from build123d import *

# Parameters (mm, degrees)
SKETCH1_W           = 150
SKETCH1_H           = 13
BOSS_EXTRUDE1_DEPTH = 40
CUT_EXTRUDE1_DEPTH  = 40
CUT_EXTRUDE3_DEPTH  = 86.988371307
SKETCH8_R           = 2
CUT_EXTRUDE7_DEPTH  = 6.5
SKETCH4_W           = 40
SKETCH4_H           = 13
CUT_EXTRUDE10_DEPTH = 77.299594056


with BuildPart() as part:
    # Sketch1 → Boss-Extrude1 (new body)
    with BuildSketch(Plane.XY):
        Rectangle(SKETCH1_W, SKETCH1_H)
    extrude(amount=BOSS_EXTRUDE1_DEPTH)

    # Sketch2 → Cut-Extrude1 (cut)
    with BuildSketch(Plane.XZ.offset(6.5)):
        Polygon((-75, 9.270509831), (-46.468304511, 0), (-75, 0), align=None)
    extrude(amount=-CUT_EXTRUDE1_DEPTH, mode=Mode.SUBTRACT)

    # Sketch3 → Cut-Extrude3 (cut, through all)
    with BuildSketch(Plane.XZ.offset(6.5)):
        Polygon((-75, 12.424896504), (-45.99315119, 3), (75, 3), (75, 40), (-75, 40), align=None)
    extrude(amount=-CUT_EXTRUDE3_DEPTH, mode=Mode.SUBTRACT)

    # Sketch8 → Cut-Extrude7 (cut)
    with BuildSketch(Plane(origin=(-4.437328231, 0, -13.656692045), x_dir=(-0.9510565162951532, 0, 0.30901699437494873), z_dir=(-0.30901699437494873, 0, -0.9510565162951532))):
        with Locations((59.193983807, 0)):
            Circle(SKETCH8_R)
    extrude(amount=-CUT_EXTRUDE7_DEPTH, mode=Mode.SUBTRACT)

    # Sketch4 → Cut-Extrude10 (cut, through all)
    with BuildSketch(Plane.XY):
        with Locations((55, 0)):
            Rectangle(SKETCH4_W, SKETCH4_H)
    extrude(amount=CUT_EXTRUDE10_DEPTH, mode=Mode.SUBTRACT)


solid = part.part
Design review of the part built by this model. Coordinates are the model's own, in mm. A direction names the side the tool comes from. Round coordinates to 2 decimals unless told otherwise and drop trailing zeros. Write each loop counter-clockwise with the first axis right and the second up, starting at its lowest first coordinate (ties: lowest second). Pieces come first, ordered by that corner, then holes.
Item 1: For faces 1 (the flat face through (-6, 0, 3)), 2 (the flat face through (-60.93, -2.98, 4.7)), list the 3-axis set-ups (+Z, -Z, +X, -X, +Y, -Y) from which the entire face can be reached by the end or side of a thin tool; tool diameter is ignored.
Item 2: For pin 1 Ø4 at (x, z) = (-57.5, 9.5) entering from +Y; pin 2 Ø6 at (x, y) = (9.5, 2.5) entering from -Z, all flat-tipped, find the tip position at first contact; note any pin that passes through.
Item 3: Consider section B-B on x = 13. Give the boundary of the cut face in (y, z), and give its area (3 significant figures).
Item 4: Consider section C-C on z = 10.5. Give the boundary of the cut face in (x, y), and give its area (3 significant figures).
Item 5: Wall thickness on L1, parallel to Z at x = 0, y = -0.25; L2, parallel to Z at x = -54, y = 4.5: over which ranges is each line inside the solid? List them lowest first.
Item 6: Consider section A-A on y = -4.5. Give the boundary of the cut face in (x, z), and give its area (3 significant figures).
Check values:
1. face 1: +Z, +X, +Y, -Y
1. face 2: -Z, -X, +Y, -Y
2. pin 1: passes through
2. pin 2: stops at z = 0
3. outline: (-6.5, 0) - (6.5, 0) - (6.5, 3) - (-6.5, 3) - close
3. area: 39.0 mm2
4. outline: (-75, -6.5) - (-69.08, -6.5) - (-69.08, 6.5) - (-75, 6.5) - close
4. area: 77.0 mm2
5. L1: z = 0 to 3
5. L2: z = 2.45 to 5.6
6. outline: (-75, 9.27) - (-46.47, 0) - (35, 0) - (35, 3) - (-45.99, 3) - (-75, 12.42) - close
6. area: 334 mm2
